from build123d import *

# Parameters (mm, degrees)
F0_R     = 55.5625
F0_R_2   = 27.0256
F1_DEPTH = 50.8
F3_R     = 31.75
F4_DEPTH = 19.05
F5_W     = 12.7
F5_H     = 33.3375
F6_DEPTH = 50.801
F7_SIZE  = 1.27
F8_D     = 10.71626
F8_DEPTH = 44.45
F8_TIP   = 3.2194893086


with BuildPart() as f1:
    # F0 (on Top) → F1 (new body)
    with BuildSketch(Plane.XY):
        Circle(F0_R)
        Circle(F0_R_2, mode=Mode.SUBTRACT)
    extrude(amount=F1_DEPTH)

    # F3 (on face) → F4 (cut)
    with BuildSketch(Plane(origin=(0, 0, 0), x_dir=(1, 0, 0), z_dir=(0, 0, -1))):
        Circle(F3_R)
    extrude(amount=-F4_DEPTH, mode=Mode.SUBTRACT)

    # F5 (on face) → F6 (cut, through all)
    with BuildSketch(Plane(origin=(0, 0, 0), x_dir=(1, 0, 0), z_dir=(0, 0, -1))):
        with Locations((0, 16.66875)):
            Rectangle(F5_W, F5_H)
    extrude(amount=-F6_DEPTH, mode=Mode.SUBTRACT)

    # F7
    f7_edges = [f1.edges().sort_by_distance(p)[0] for p in [
        (-55.5625, 0, 50.8),
        (-55.5625, 0, 0),
    ]]
    chamfer(f7_edges, length=F7_SIZE)

    # F8
    with Locations(Plane(origin=(0, 0, 0), x_dir=(1, 0, 0), z_dir=(0, 0, -1))):
        with Locations((-31.4308964237, -31.4308964237), (-31.4308964237, 31.4308964237), (31.4308964237, 31.4308964237), (31.4308964237, -31.4308964237)):
            Hole(F8_D / 2, depth=F8_DEPTH)
            with Locations((0, 0, -(F8_DEPTH + F8_TIP / 2))):  # 118° drill point
                Cone(0, F8_D / 2, F8_TIP, mode=Mode.SUBTRACT)


solid = f1.part
Geometry: final body of the model. Coordinates: model frame, mm. A direction names the side the tool comes from. Give positions to 0.01 mm unless a question says otherwise; leave off trailing zeros. Loops run counter-clockwise (first coordinate to the right, second up) from the corner with the lowest first, then second, coordinate; pieces in that order, holes last. Notation, with made-up numbers: (32, -2) -> (69, -2) arc R21 cw to (69, 35) -> close; hole circle Ø3 at (50, -37.5). An arc over 180 degrees is marked (long way). Put each result on its own line as item: value.
1. Ray query, line 1 along X through (y, z) = (-35.5, 30); line 2 along X through (y, z) = (21, 7.5); line 3 along Y through (x, z) = (0, 30.5). Return the intervals inside material, ascending. Write a range as [from, to].
Taken from the geometry:
line 1: x = [-42.74, -34.92], [-27.94, 27.94], [34.92, 42.74]
line 2: x = [-51.44, -23.81], [23.81, 51.44]
line 3: y = [-55.56, -33.34], [27.03, 55.56]
2. Pin query (flat end, axial travel): P1, Ø4, axis at y = -28, z = 6, coming from the +X side; P2, Ø1.5, axis at x = 22, z = 34, coming from the -Y side; P3, Ø3.5, axis at y = -29, z = 25.5, coming from the +X side. Return the tip coordinate at first contact, or that it passes through.
Taken from the geometry:
P1: stops at x = 49.1
P2: stops at y = -51.34
P3: stops at x = 48.42
3. Set-up query: faces 1 (the cylindrical face through (-27.18, -28.17, 22.54)), 2 (the flat face through (0, -33.338, 25)), 3 (the flat face through (23, -23, 0)). Return all of +Z, -Z, +X, -X, +Y, -Y with unobstructed straight access to the full face (end or side cutting, diameter ignored); none if empty.
Taken from the geometry:
face 1: -Z
face 2: +Z, -Z
face 3: -Z, +X, -X, +Y, -Y
4. Cut plane C-C (z = 35). Count the separate pieces of the cut face and the enclosed holes in it, plus the area to 3 significant figures.
Taken from the geometry:
separate pieces: 1
enclosed holes: 5
area: 6,960 mm2
5. Pull-direction query (Y, two-part tool) for faces 4 (the conical face through (31.93, -32.22, 47.11)), 5 (the cylindrical face through (-7.23, 55.09, 25.06)), 6 (the flat face through (11, 25, 50.8)); classes: released by +Y, released by -Y, zero draft, split by the parting line, or undercut.
Taken from the geometry:
face 4: undercut
face 5: split by the parting line
face 6: zero draft
6. Cut plane B-B (x = 0). Return the cut outline in (y, z).
Taken from the geometry:
outline: (-55.56, 1.27) -> (-54.29, 0) -> (-33.34, 0) -> (-33.34, 50.8) -> (-54.29, 50.8) -> (-55.56, 49.53) -> close; (27.03, 19.05) -> (31.75, 19.05) -> (31.75, 0) -> (54.29, 0) -> (55.56, 1.27) -> (55.56, 49.53) -> (54.29, 50.8) -> (27.03, 50.8) -> close
7. Cut plane A-A (y = 0). Return the cut outline in (x, z).
Taken from the geometry:
outline: (-55.56, 1.27) -> (-54.29, 0) -> (-31.75, 0) -> (-31.75, 19.05) -> (-27.03, 19.05) -> (-27.03, 50.8) -> (-54.29, 50.8) -> (-55.56, 49.53) -> close; (27.03, 19.05) -> (31.75, 19.05) -> (31.75, 0) -> (54.29, 0) -> (55.56, 1.27) -> (55.56, 49.53) -> (54.29, 50.8) -> (27.03, 50.8) -> close
